For this review, take the finished solid that the model builds, in its own axes (mm). Face numbers are marked on the shaded views. A direction names the side the tool comes from. Coordinates: 2 decimals unless noted, no trailing zeros. Write each loop counter-clockwise with the first axis right and the second up, starting at its lowest first coordinate (ties: lowest second). Pieces come first, ordered by that corner, then holes.
1) We need section A-A on y = 0. Write out the cut boundary in (x, z).
2) We need section B-B on x = -24. Write out the cut boundary in (y, z), then the cut area to 3 significant figures.
3) For the marked faces 5 and 6, list the 3-axis set-ups (+Z, -Z, +X, -X, +Y, -Y) from which the entire face can be reached by the end or side of a thin tool; tool diameter is ignored.
4) To check wall thickness, follow line 1 along Y through (x, z) = (-51.5, 85); line 2 along X through (y, z) = (53.5, 169); line 3 along Z through (x, y) = (-89, 61.5). State the ranges of each line that lie inside material, in increasing order.
5) Mouldability with a two-part tool opening along Y and no side actions: class the marked faces 1, 2, 3 and 4 as pulls with the +Y half, pulls with the -Y half, needs draft (parallel to the pull), parting line crosses it, or undercut.
6) We need section D-D on z = 128.5. Write out the cut boundary in (x, y), then the cut area to 3 significant figures.
7) Insertion check: P1, Ø15, axis at x = -93.5, y = -7.5, coming from the +Z side; P2, Ø18, axis at y = 5, z = 144, coming from the -X side; P3, Ø3, axis at x = -63, z = 95.5, coming from the -Y side. Each pin has a flat end and moves straight along its axis. Give the tip position at first contact, or say it passes through.
8) We need section C-C on y = 28.5. Write out the cut boundary in (x, z).
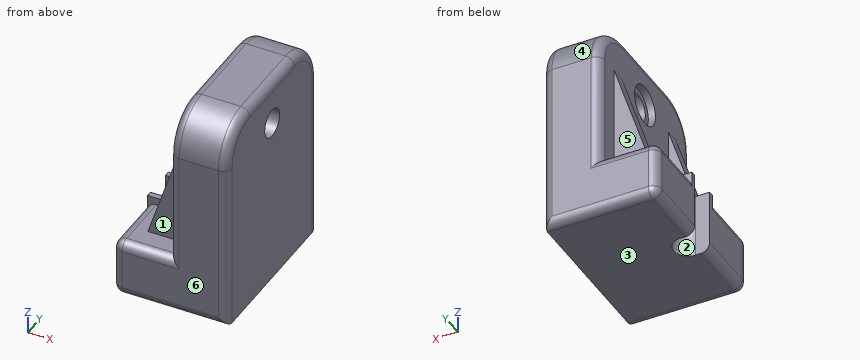
from build123d import *

# Parameters (mm, degrees)
F1_DEPTH  = 76.2
F2_R      = 12.7
F3_DEPTH  = 101.601
F5_DEPTH  = 50.801
F6_R      = 38.1
F7_R      = 17.78
F7_R_2    = 12.7
F8_DEPTH  = 6.35
F12_DEPTH = 6.35
F15_DEPTH = 6.35
F16_R     = 7.971733183


# Not quite as in the source:
# - a pattern or mirror of a feature is missing from the dataset's text; its kind, count and spacing are read off the source's solid


with BuildPart() as f1:
    # F0 (on Front) → F1 (new body, symmetric)
    with BuildSketch(Plane.XZ):
        Polygon((-101.6, 0), (0, 0), (0, 188.9744497656), (-50.8, 188.9744497656), (-50.8, 50.8), (-101.6, 50.8), align=None)
    extrude(amount=F1_DEPTH, both=True)

    # F2 (on face) → F3 (cut, through all)
    with BuildSketch(Plane.YZ):
        with Locations((0, 150.8744497656)):
            Circle(F2_R)
    extrude(amount=-F3_DEPTH, mode=Mode.SUBTRACT)

    # F4 (on face) → F5 (cut, through all)
    with BuildSketch(Plane.XY.offset(50.8)):
        with BuildLine():
            Line((-88.9, 12.7), (-101.6, 12.7))
            Line((-101.6, 12.7), (-101.6, -12.7))
            Line((-101.6, -12.7), (-88.9, -12.7))
            ThreePointArc((-88.9, -12.7), (-76.2, 0), (-88.9, 12.7))
        make_face()
    extrude(amount=-F5_DEPTH, mode=Mode.SUBTRACT)

    # F6
    f6_edges = [f1.edges().sort_by_distance(p)[0] for p in [
        (-25.4, -76.2, 188.97445),
        (-25.4, 76.2, 188.97445),
    ]]
    fillet(f6_edges, radius=F6_R)

    # F7 (on face) → F8 (cut)
    with BuildSketch(Plane(origin=(-50.8, 0, 0), x_dir=(0, -1, 0), z_dir=(-1, 0, 0))):
        with Locations((0, 150.8744497656)):
            Circle(F7_R)
        with Locations((0, 150.8744497656)):
            Circle(F7_R_2, mode=Mode.SUBTRACT)
    extrude(amount=-F8_DEPTH, mode=Mode.SUBTRACT)

    # F11 (on offset) → F12 (join, symmetric)
    with BuildSketch(Plane.XZ.offset(45.974)):
        Polygon((-83.1002444029, 50.8), (-50.8, 50.8), (-50.8, 150.8744497656), align=None)
    f12 = extrude(amount=F12_DEPTH, both=True)

    # F12_copies: F12 across plane
    add(f12.mirror(Plane.ZX))

    # F14 (on face) → F15 (join)
    with BuildSketch(Plane.XY.offset(50.8)):
        with BuildLine():
            Line((-101.6, -12.7), (-101.6, -17.5260007381))
            Line((-101.6, -17.5260007381), (-88.9, -17.5260007381))
            ThreePointArc((-88.9, -17.5260007381), (-71.3739992619, 0), (-88.9, 17.5260007381))
            Line((-88.9, 17.5260007381), (-101.6, 17.5260007381))
            Line((-101.6, 17.5260007381), (-101.6, 12.7))
            Line((-101.6, 12.7), (-88.9, 12.7))
            ThreePointArc((-88.9, 12.7), (-76.2, 0), (-88.9, -12.7))
            Line((-88.9, -12.7), (-101.6, -12.7))
        make_face()
    extrude(amount=F15_DEPTH)

    # F16
    f16_edges = [f1.edges().sort_by_distance(p)[0] for p in [
        (-76.2, -76.2, 50.8),
        (-76.2, 76.2, 50.8),
        (-50.8, -76.2, 0),
        (0, -76.2, 75.437225),
        (-25.4, -76.2, 150.87445),
        (-50.8, -76.2, 100.837225),
        (-101.6, -76.2, 25.4),
        (-50.8, 76.2, 0),
        (-101.6, 76.2, 25.4),
        (-101.6, 46.863, 50.8),
        (-101.6, -46.863, 50.8),
        (-101.6, -44.45, 0),
        (-101.6, 44.45, 0),
        (0, 76.2, 75.437225),
        (-50.8, 76.2, 100.837225),
        (0, 65.040768, 177.815218),
        (-50.8, 65.040768, 177.815218),
        (0, 0, 188.97445),
        (-50.8, 0, 188.97445),
        (-50.8, -65.040768, 177.815218),
        (0, -65.040768, 177.815218),
    ]]
    fillet(f16_edges, radius=F16_R)


solid = f1.part
Result:
1. outline: (-76.2, 0) - (0, 0) - (0, 138.17) - (-44.45, 138.17) - (-44.45, 133.09) - (-50.8, 133.09) - (-50.8, 50.8) - (-71.37, 50.8) - (-71.37, 57.15) - (-76.2, 57.15) - close; (-50.8, 168.65) - (-44.45, 168.65) - (-44.45, 163.57) - (0, 163.57) - (0, 181) arc R7.97 ccw to (-7.97, 188.97) - (-42.83, 188.97) arc R7.97 ccw to (-50.8, 181) - close
2. outline: (-76.2, 7.97) arc R7.97 ccw to (-68.23, 0) - (68.23, 0) arc R7.97 ccw to (76.2, 7.97) - (76.2, 150.87) arc R38.1 ccw to (38.1, 188.97) - (-38.1, 188.97) arc R38.1 ccw to (-76.2, 150.87) - close; hole circle Ø25.4 at (0, 150.87)
2. area: 27,600 mm2
3. face 5: +Z, -X, +Y
3. face 6: +Z, -Z, +X, -X, -Y
4. line 1: y = -52.32 to -39.62, 39.62 to 52.32
4. line 2: x = -50.8 to 0
4. line 3: z = 0 to 50.8
5. face 1: pulls with the -Y half
5. face 2: undercut
5. face 3: needs draft
5. face 4: pulls with the +Y half
6. outline: (-58.02, -52.32) - (-50.8, -52.32) - (-50.8, -68.23) arc R7.97 ccw to (-42.83, -76.2) - (-7.97, -76.2) arc R7.97 ccw to (0, -68.23) - (0, 68.23) arc R7.97 ccw to (-7.97, 76.2) - (-42.83, 76.2) arc R7.97 ccw to (-50.8, 68.23) - (-50.8, 52.32) - (-58.02, 52.32) - (-58.02, 39.62) - (-50.8, 39.62) - (-50.8, -39.62) - (-58.02, -39.62) - close
6. area: 7,870 mm2
7. P1: stops at z = 57.15
7. P2: stops at x = -44.45
7. P3: stops at y = -52.32
8. outline: (-101.6, 7.97) arc R7.97 ccw to (-93.63, 0) - (0, 0) - (0, 181) arc R7.97 ccw to (-7.97, 188.97) - (-42.83, 188.97) arc R7.97 ccw to (-50.8, 181) - (-50.8, 50.8) - (-93.63, 50.8) arc R7.97 ccw to (-101.6, 42.83) - close
